Verification items for the finished model (mm, model axes). A direction names the side the tool comes from. Give positions to 0.01 mm unless a question says otherwise; leave off trailing zeros. Loops run counter-clockwise (first coordinate to the right, second up) from the corner with the lowest first, then second, coordinate; pieces in that order, holes last. Notation, with made-up numbers: (36.5, 89.5) - (41.5, 89.5) arc R19 cw to (41.5, 111.5) - close; hole circle Ø2 at (0, 38.25). An arc over 180 degrees is marked (long way). One line per item, written item: value. Start each with the question number.
1. Sectioned sample at B-B (x = 3). Record the cut outline in (y, z), plus the area to 3 significant figures.
2. Sectioned sample at C-C (y = -5.5). Record the cut outline in (x, z).
3. Access from +Z, -Z, +X, -X, +Y, -Y to the whole of each face (thin tool, end or side, straight path). Record for faces 1 (the flat face through (-5, 6, 6)), 2 (the flat face through (-7, 8, 6)), 3 (the flat face through (5, -7, 6)).
4. Gauge pin test, flat end, axial feed: pin 1 (0.9 mm diameter, centred on y = -6.5, z = 6, fed in from -X). Record the tip position at first contact, or that the pin passes through.
5. Scan lines: L1, parallel to Y at x = 5.5, z = 6.7; L2, parallel to Y at x = 4, z = 5.2; L3, parallel to X at y = 5.25, z = 6.15. Record each from-to range of solid material in increasing order. Write a range as [from, to].
6. Sectioned sample at A-A (z = 6.8). Record the cut outline in (x, y).
from build123d import *

# Parameters (mm, degrees)
F3_W     = 3
F3_H     = 5
F3_H_2   = 3
F4_DEPTH = 3


with BuildPart() as f4:
    # F3 (on face) → F4 (new body)
    with BuildSketch(Plane.XY.offset(5)):
        Polygon((-5, 0), (-5, -5), (0, -5), (5, -5), (5, 0), (5, 5), (0, 5), (-5, 5), align=None)
        with Locations((-6.5, 2.5)):
            Rectangle(F3_W, F3_H)
        with Locations((-6.5, 6.5)):
            Rectangle(F3_W, F3_H_2)
        with Locations((6.5, -2.5)):
            Rectangle(F3_W, F3_H)
        with Locations((6.5, -6.5)):
            Rectangle(F3_W, F3_H_2)
        with Locations((-6.5, -2.5)):
            Rectangle(F3_W, F3_H)
        with Locations((6.5, 2.5)):
            Rectangle(F3_W, F3_H)
    extrude(amount=F4_DEPTH)


solid = f4.part
Results are:
1. outline: (-5, 5) - (5, 5) - (5, 8) - (-5, 8) - close
1. area: 30.0 mm^2
2. outline: (5, 5) - (8, 5) - (8, 8) - (5, 8) - close
3. face 1: +Z, -Z, +X, +Y
3. face 2: +Z, -Z, +X, -X, +Y
3. face 3: +Z, -Z, -X, -Y
4. pin 1: stops at x = 5
5. L1: y = [-8, 5]
5. L2: y = [-5, 5]
5. L3: x = [-8, -5]
6. outline: (-8, -5) - (5, -5) - (5, -8) - (8, -8) - (8, 5) - (-5, 5) - (-5, 8) - (-8, 8) - close
